Design review of the part built by this model. Coordinates are the model's own, in mm. A direction names the side the tool comes from. Coordinates: 2 decimals unless noted, no trailing zeros. Write each loop counter-clockwise with the first axis right and the second up, starting at its lowest first coordinate (ties: lowest second). Pieces come first, ordered by that corner, then holes. Notation, with made-up numbers: (-33.5, 29.25) - (-11.5, 29.25) arc R33 ccw to (-11.5, 57.25) - close; hole circle Ø7 at (38.25, 88.25). An arc over 180 degrees is marked (long way). Answer as a JSON object with one key per item and string values.
```python
from build123d import *

# Parameters (mm, degrees)
SKETCH_1_W      = 60
SKETCH_1_H      = 36
SKETCH_1_W_2    = 35
SKETCH_1_H_2    = 4
EXTRUDE_1_DEPTH = 2
SKETCH_2_W      = 60
SKETCH_2_H      = 36
SKETCH_2_W_2    = 56
SKETCH_2_H_2    = 32
EXTRUDE_2_DEPTH = 2


with BuildPart() as part:
    # ｽｹｯﾁ1 → ﾎﾞｽ - 押し出し1 (new body)
    with BuildSketch(Plane.XY):
        Rectangle(SKETCH_1_W, SKETCH_1_H)
        with Locations((0, 14)):
            Rectangle(SKETCH_1_W_2, SKETCH_1_H_2, mode=Mode.SUBTRACT)
    extrude(amount=EXTRUDE_1_DEPTH)

    # ｽｹｯﾁ2 → ﾎﾞｽ - 押し出し2 (add)
    with BuildSketch(Plane.XY.offset(2)):
        Rectangle(SKETCH_2_W, SKETCH_2_H)
        Rectangle(SKETCH_2_W_2, SKETCH_2_H_2, mode=Mode.SUBTRACT)
    extrude(amount=EXTRUDE_2_DEPTH)


solid = part.part
```
(1) To check wall thickness, follow line 1 (Y direction, x = -1.5, z = 1.9); line 2 (X direction, y = 14.5, z = 0.8); line 3 (X direction, y = -6.5, z = 3.65). State the ranges of each line that lie inside material, in increasing order. Write a range as from..to.
Solved:
{"line 1": "y = -18..12, 16..18", "line 2": "x = -30..-17.5, 17.5..30", "line 3": "x = -30..-28, 28..30"}
(2) Take a section at A-A, the plane z = 0.85. Write out the cut boundary in (x, y), and give its area (3 significant figures).
Solved:
{"outline": "(-30, -18) - (30, -18) - (30, 18) - (-30, 18) - close; hole (-17.5, 12) - (17.5, 12) - (17.5, 16) - (-17.5, 16) - close", "area": "2,020 mm^2"}
(3) Tool access review of faces 4 (the face through (0, -18, 2)), 5 (the face through (0, 16, 2)), 6 (the face through (17.5, 14, 1)): name each direction out of +Z, -Z, +X, -X, +Y, -Y from which nothing blocks a thin tool from reaching the whole face with its end or side.
Solved:
{"face 4": "+Z, -Z, +X, -X, -Y", "face 5": "+Z", "face 6": "+Z, -Z"}
(4) Take a section at B-B, the plane x = -8. Write out the cut boundary in (y, z).
Solved:
{"outline": "(-18, 0) - (12, 0) - (12, 2) - (-16, 2) - (-16, 4) - (-18, 4) - close; (16, 0) - (18, 0) - (18, 4) - (16, 4) - close"}
(5) Take a section at C-C, the plane y = 14. Write out the cut boundary in (x, z).
Solved:
{"outline": "(-30, 0) - (-17.5, 0) - (-17.5, 2) - (-28, 2) - (-28, 4) - (-30, 4) - close; (17.5, 0) - (30, 0) - (30, 4) - (28, 4) - (28, 2) - (17.5, 2) - close"}
(6) Take a section at D-D, the plane y = -10. Write out the cut boundary in (x, z).
Solved:
{"outline": "(-30, 0) - (30, 0) - (30, 4) - (28, 4) - (28, 2) - (-28, 2) - (-28, 4) - (-30, 4) - close"}
(7) The part is to be moulded in two halves that separate along X. For faces 1 (the face through (28, 0, 3)), 2 (the face through (30, 0, 2)), 3 (the face through (0, 0, 0)), say which applies: pulls with the +X half, pulls with the -X half, needs draft (parallel to the pull), parting line crosses it, or undercut.
Solved:
{"face 1": "undercut", "face 2": "pulls with the +X half", "face 3": "needs draft"}
(8) For pin 1 (8 mm diameter, centred on x = -6, y = -5, fed in from -Z); pin 2 (10 mm diameter, centred on x = -1, y = -2, fed in from +Z), all flat-tipped, find the tip position at first contact; note any pin that passes through.
Solved:
{"pin 1": "stops at z = 0", "pin 2": "stops at z = 2"}
